Check sheet for the modelled part. Datum: model origin and axes. Units: mm. Give positions to 0.01 mm unless a question says otherwise; leave off trailing zeros. Loops run counter-clockwise (first coordinate to the right, second up) from the corner with the lowest first, then second, coordinate; pieces in that order, holes last. Notation, with made-up numbers: (89, -6) -> (93, -6) arc R10 ccw to (93, 1) -> close; hole circle Ø5 at (89, -11). An arc over 180 degrees is marked (long way). Answer as CSV lines item,"result". Start each with the question number.
(1) Section check D-D on x = -1.75. Enter the section's corners in (y, z).
(2) Section check C-C on y = 0.3. Enter the section's corners in (x, z), plus the area to 3 significant figures.
(3) Section check A-A on x = 0. Enter the section's corners in (y, z).
(4) Material ranges on line 1 (Y direction, x = 0, z = 2.95); line 2 (X direction, y = 0.1, z = 4.6); line 3 (X direction, y = -1.3, z = 1.05), recorded low to high. Write a range as from..to.
(5) Gauge pin test, flat end, axial feed: pin 1 Ø1.5 at (x, y) = (0, 0) entering from -Z. Record the tip position at first contact, or that the pin passes through.
(6) Section check B-B on z = 0.3. Enter the section's corners in (x, y).
from build123d import *

# Parameters (mm, degrees)
F1_DEPTH = 5
F2_COUNT = 6
F2_ANGLE = 300
F3_R     = 1.6
F4_DEPTH = 5.001


with BuildPart() as f1:
    # F0 (on Top) → F1 (new body)
    with BuildSketch(Plane.XY):
        Polygon((-1.443376, 2.5), (0, 0), (1.443376, 2.5), align=None)
    extrude(amount=F1_DEPTH)

    # F2: F1 ×6 about axis
    f2_axis = Axis((0, 0, 2.5), (0, 0, 1))


with BuildPart() as f1_1:
    add(f1.part)
    for i in range(1, F2_COUNT):
        add(f1.part.rotate(f2_axis, i * F2_ANGLE / (F2_COUNT - 1)))

    # F3 (on face) → F4 (cut, through all)
    with BuildSketch(Plane.XY.offset(5)):
        Circle(F3_R)
    extrude(amount=-F4_DEPTH, mode=Mode.SUBTRACT)


solid = f1_1.part
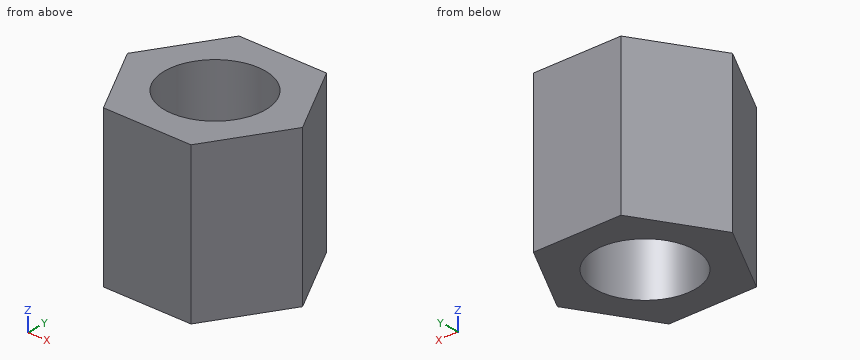
Working result:
1,outline,"(-1.97, 0) -> (1.97, 0) -> (1.97, 5) -> (-1.97, 5) -> close"
2,outline,"(-2.71, 0) -> (-1.57, 0) -> (-1.57, 5) -> (-2.71, 5) -> close; (1.57, 0) -> (2.71, 0) -> (2.71, 5) -> (1.57, 5) -> close"
2,area,"11.4 mm^2"
3,outline,"(-2.5, 0) -> (-1.6, 0) -> (-1.6, 5) -> (-2.5, 5) -> close; (1.6, 0) -> (2.5, 0) -> (2.5, 5) -> (1.6, 5) -> close"
4,line 1,"y = -2.5..-1.6, 1.6..2.5"
4,line 2,"x = -2.83..-1.6, 1.6..2.83"
4,line 3,"x = -2.14..-0.93, 0.93..2.14"
5,pin 1,"passes through"
6,outline,"(-2.89, 0) -> (-1.44, -2.5) -> (1.44, -2.5) -> (2.89, 0) -> (1.44, 2.5) -> (-1.44, 2.5) -> close; hole circle Ø3.2 at (0, 0)"
